Geometry: final body of the model. Coordinates: model frame, mm. Face numbers are marked on the shaded views. A direction names the side the tool comes from. Coordinates: 2 decimals unless noted, no trailing zeros. Order: outer loops, then holes, each group sorted by start corner. A loop starts at its lowest first (then second) coordinate and runs counter-clockwise, first axis right, second up. Notation, with made-up numbers: M 26.25,-34 L 56.25,-34 A29 ccw 56.25,1 Z; hole C 39,20.25 d3. An arc over 180 degrees is marked long. Write item = value, one per line.
from build123d import *

# Parameters (mm, degrees)
F0_R     = 7.9375
F1_DEPTH = 50.8
F2_R     = 7.9375
F3_DEPTH = 50.8


with BuildPart() as f1:
    # F0 (on Front) → F1 (new body, symmetric)
    with BuildSketch(Plane.XZ):
        Polygon((-38.1, -32.143515), (-38.1, -38.1), (38.1, -38.1), (38.1, -32.143515), (16.356649, -19.013904), (38.1, -5.884292), (38.1, 0), (31.75, 0), (31.75, 6.35), (38.1, 6.35), (38.1, 38.1), (0, 0), (-38.1, 38.1), (-38.1, 6.35), (-31.75, 6.35), (-31.75, 0), (-38.1, 0), (-38.1, -5.884292), (-16.356649, -19.013904), align=None)
        with Locations((0, -20.482006)):
            Circle(F0_R, mode=Mode.SUBTRACT)
    extrude(amount=F1_DEPTH, both=True)

    # F2 (on Top) → F3 (cut, symmetric)
    with BuildSketch(Plane.XY):
        Circle(F2_R)
    extrude(amount=F3_DEPTH, both=True, mode=Mode.SUBTRACT)


solid = f1.part
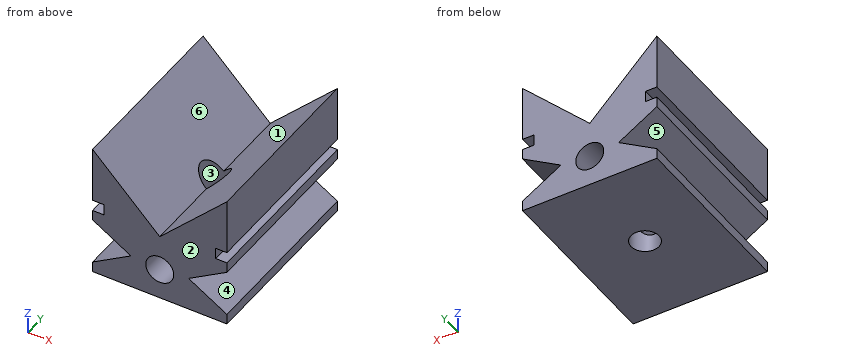
1) Section A-A, the plane x = 30.5. Return loops of the section in (y, z).
Numbers:
outline = M -50.8,-38.1 L 50.8,-38.1 L 50.8,-27.55 L -50.8,-27.55 Z; M -50.8,-10.47 L 50.8,-10.47 L 50.8,30.5 L -50.8,30.5 Z
2) Line query: L1, parallel to Y at x = 0, z = -8; L2, parallel to X at y = 0.5, z = -3; L3, parallel to Z at x = -23, y = 3.5. Output: solid intervals per line, ascending.
Numbers:
L1 = -50.8 to -7.94, 7.94 to 50.8
L2 = -38.1 to -7.92, 7.92 to 38.1
L3 = -38.1 to -23.03, -15 to 23
3) Pin query (flat end, axial travel): pin 1 (12 mm diameter, centred on y = 9.5, z = -24, fed in from +X); pin 2 (9.5 mm diameter, centred on x = 0, y = 0, fed in from +Z); pin 3 (2 mm diameter, centred on y = 23.5, z = -30, fed in from -X); pin 4 (3 mm diameter, centred on x = 34, y = 2.5, fed in from +Z). Return the tip coordinate at first contact, or that it passes through.
Numbers:
pin_1 = 34.55
pin_2 = through
pin_3 = -36.21
pin_4 = 35.5
4) Section C-C, the plane z = -17. Return loops of the section in (x, y) (1 decimal), and give its area (3 significant figures).
Numbers:
outline = M -19.7,-50.8 L -7.1,-50.8 L -7.1,-3.5 A7.9 cw -7.1,3.5 L -7.1,50.8 L -19.7,50.8 Z; M 7.1,-50.8 L 19.7,-50.8 L 19.7,50.8 L 7.1,50.8 L 7.1,3.5 A7.9 cw 7.1,-3.5 Z
area = 2,540 mm²
5) Set-up query: the marked faces 4, 5 and 6. Return all of +Z, -Z, +X, -X, +Y, -Y with unobstructed straight access to the full face (end or side cutting, diameter ignored); none if empty.
Numbers:
face_4 = +X, +Y, -Y
face_5 = -X, +Y, -Y
face_6 = +Z, +Y, -Y
6) Mould query, pull axis Y, two halves, no side actions, for the marked faces 1, 2 and 3. Classes: pulls with the +Y half, pulls with the -Y half, needs draft (parallel to the pull), parting line crosses it, or undercut.
Numbers:
face_1 = needs draft
face_2 = pulls with the -Y half
face_3 = undercut
